```python
from build123d import *

# Parameters (mm, degrees)
BOSS_EXTRUDE1_DEPTH                             = 14
CUT_EXTRUDE1_DEPTH                              = 17.760296299
CUT_EXTRUDE1_DEPTH_BACK                         = 0.2
SKETCH4_R                                       = 3.25
CSK_FOR_M3_FLAT_HEAD_MACHINE_SCREW4_D           = 3.6
CSK_FOR_M3_FLAT_HEAD_MACHINE_SCREW4_DEPTH       = 7.5
CSK_FOR_M3_FLAT_HEAD_MACHINE_SCREW4_CSINK_D     = 6.3
CSK_FOR_M3_FLAT_HEAD_MACHINE_SCREW4_CSINK_ANGLE = 90
CSK_FOR_M3_FLAT_HEAD_MACHINE_SCREW4_TIP         = 1.081549114


with BuildPart() as part:
    # Sketch1 → Boss-Extrude1 (new body)
    with BuildSketch(Plane(origin=(0, 0, 0), x_dir=(1, 0, 0), z_dir=(0, 1, 0))):
        with BuildLine():
            Line((-5, -7.486681333), (5, -7.486681333))
            Line((5, -7.486681333), (3.845299462, -5.486681333))
            ThreePointArc((3.845299462, -5.486681333), (6.363430853, -2.096842336), (6.35376849, 2.125941198))
            Line((6.35376849, 2.125941198), (3.982959352, 1.332679557))
            ThreePointArc((3.982959352, 1.332679557), (0, -4.2), (-3.982959352, 1.332679557))
            Line((-3.982959352, 1.332679557), (-6.35376849, 2.125941198))
            ThreePointArc((-6.35376849, 2.125941198), (-6.363430853, -2.096842336), (-3.845299462, -5.486681333))
            Line((-3.845299462, -5.486681333), (-5, -7.486681333))
        make_face()
    extrude(amount=BOSS_EXTRUDE1_DEPTH)

    # Sketch4 → Cut-Extrude1 (cut, two sides: drawn at the far end of the back side and taken through both)
    with BuildSketch(Plane(origin=(0, 0, 4.2), x_dir=(-1, 0, 0), z_dir=(0, 0, -1)).offset(-CUT_EXTRUDE1_DEPTH_BACK)):
        with Locations((0, 7)):
            Circle(SKETCH4_R)
    extrude(amount=CUT_EXTRUDE1_DEPTH + CUT_EXTRUDE1_DEPTH_BACK, mode=Mode.SUBTRACT)

    # CSK for M3 Flat Head Machine Screw4
    with Locations(Plane(origin=(0, 0, 4.4), x_dir=(-1, 0, 0), z_dir=(0, 0, -1))):
        with Locations((0, 7)):
            CounterSinkHole(CSK_FOR_M3_FLAT_HEAD_MACHINE_SCREW4_D / 2, CSK_FOR_M3_FLAT_HEAD_MACHINE_SCREW4_CSINK_D / 2, depth=CSK_FOR_M3_FLAT_HEAD_MACHINE_SCREW4_DEPTH, counter_sink_angle=CSK_FOR_M3_FLAT_HEAD_MACHINE_SCREW4_CSINK_ANGLE)
            with Locations((0, 0, -(CSK_FOR_M3_FLAT_HEAD_MACHINE_SCREW4_DEPTH + CSK_FOR_M3_FLAT_HEAD_MACHINE_SCREW4_TIP / 2))):  # 118° drill point
                Cone(0, CSK_FOR_M3_FLAT_HEAD_MACHINE_SCREW4_D / 2, CSK_FOR_M3_FLAT_HEAD_MACHINE_SCREW4_TIP, mode=Mode.SUBTRACT)


solid = part.part
```
Check sheet for the modelled part. Datum: model origin and axes. Units: mm. A direction names the side the tool comes from. Give positions to 0.01 mm unless a question says otherwise; leave off trailing zeros. Write each loop counter-clockwise with the first axis right and the second up, starting at its lowest first coordinate (ties: lowest second). Pieces come first, ordered by that corner, then holes.
Item 1: Cross-section at A-A (x = 0). Enter the section's corners in (y, z), and give its area (3 significant figures).
Item 2: Scan lines: L1, parallel to Y at x = 0, z = 6.7; L2, parallel to X at y = 7, z = 0; L3, parallel to X at y = 7, z = 3.75. Record each from-to range of solid material in increasing order.
Item 3: Cross-section at B-B (y = 7). Enter the section's corners in (x, z).
Item 4: Gauge pin test, flat ends, axial feed: pin 1 (1 mm diameter, centred on y = 5.5, z = 2, fed in from +X); pin 2 (2 mm diameter, centred on y = 10, z = 2, fed in from +X); pin 3 (8 mm diameter, centred on x = 1.5, y = 5, fed in from -Z). Record the tip position at first contact, or that the pin passes through.
Item 5: Draft check along Z on faces 6 (the face through (0, 0, 5)), 7 (the face through (6.344, 6.902, 2.154)), 8 (the face through (5.185, 6.902, -1.735)). Enter one of: released by +Z, released by -Z, zero draft, split by the parting line, or undercut.
Item 6: Cross-section at D-D (z = 4.75). Enter the section's corners in (x, y).
Item 7: Cross-section at C-C (z = 0). Enter the section's corners in (x, y), and give its area (3 significant figures).
Item 8: Access from +Z, -Z, +X, -X, +Y, -Y to the whole of each face (thin tool, end or side, straight path). Record for faces 1 (the face through (4.43, 6.9, 6.5)), 2 (the face through (-5.152, 6.902, -1.724)), 3 (the face through (0, 14, 5)), 4 (the face through (-4.415, 6.902, 6.473)), 5 (the face through (-3.002, 5.755, 3.736)).
Report:
1. outline: (0, 4.2) - (3.75, 4.2) - (3.75, 4.4) - (3.85, 4.4) - (5.2, 5.75) - (5.2, 7.49) - (0, 7.49) - close; (8.8, 5.75) - (10.15, 4.4) - (10.25, 4.4) - (10.25, 4.2) - (14, 4.2) - (14, 7.49) - (8.8, 7.49) - close
1. area: 31.8 mm2
2. L1: y = 0 to 5.2, 8.8 to 14
2. L2: x = -6.7 to -4.2, 4.2 to 6.7
2. L3: x = -5.55 to -3.25, 3.25 to 5.55
3. outline: (-6.35, -2.13) - (-3.98, -1.33) arc R4.2 cw to (-3.25, 2.66) - (-3.25, 4.4) - (-3.15, 4.4) - (-1.8, 5.75) - (-1.8, 7.49) - (-5, 7.49) - (-3.85, 5.49) arc R6.7 ccw to start; (1.8, 5.75) - (3.15, 4.4) - (3.25, 4.4) - (3.25, 2.66) arc R4.2 cw to (3.98, -1.33) - (6.35, -2.13) arc R6.7 ccw to (3.85, 5.49) - (5, 7.49) - (1.8, 7.49) - close
4. pin 1: stops at x = 6.53
4. pin 2: stops at x = 6.62
4. pin 3: stops at z = -1.84
5. face 6: zero draft
5. face 7: undercut
5. face 8: released by -Z
6. outline: (-4.73, 0) - (4.73, 0) - (4.73, 14) - (-4.73, 14) - close; hole circle Ø5.6 at (0, 7)
7. outline: (-6.7, 0) - (-4.2, 0) - (-4.2, 14) - (-6.7, 14) - close; (4.2, 0) - (6.7, 0) - (6.7, 14) - (4.2, 14) - close
7. area: 70.0 mm2
8. face 1: +X, +Y, -Y
8. face 2: -Z, +Y, -Y
8. face 3: +Z, -Z, +X, -X, +Y
8. face 4: -X, +Y, -Y
8. face 5: -Z
